from build123d import *

# Parameters (mm, degrees)
SKETCH_2_R               = 7.5
CUT_EXTRUDE_1_DEPTH      = 134.542128184
CUT_EXTRUDE_2_DEPTH      = 134.542128184
PATTERN_CIRCULAR_1_COUNT = 6
FILLET_1_R               = 2.5
SKETCH_4_R               = 100
SKETCH_4_R_2             = 72.5
CUT_EXTRUDE_3_DEPTH      = 20


with BuildPart() as part:
    # 草图1 → 旋转1 (revolve)
    with BuildSketch(Plane(origin=(0, 0, 0), x_dir=(0, 0, -1), z_dir=(1, 0, 0)), mode=Mode.PRIVATE) as revolve_1_sk:
        Polygon((-91.5, 33), (-91.5, 0), (-65, 0), (-65, 3), (-65, 33), (-69, 33), align=None)
    revolve(revolve_1_sk.sketch.rotate(Axis((0, 0, 0), (0, 1, 0)), 180), axis=Axis((0, 0, 0), (0, 1, 0)))

    # 草图2 → 切除-拉伸1 (cut, through all)
    with BuildSketch(Plane(origin=(0, 33, 0), x_dir=(1, 0, 0), z_dir=(0, 1, 0))):
        with Locations(Location((0, 80, 0), (0, 0, 270))):
            Circle(SKETCH_2_R)
    cut_extrude_1 = extrude(amount=-CUT_EXTRUDE_1_DEPTH, mode=Mode.SUBTRACT)

    # 草图3 → 切除-拉伸2 (cut, through all)
    with BuildSketch(Plane(origin=(0, 33, 0), x_dir=(1, 0, 0), z_dir=(0, 1, 0))):
        with BuildLine():
            Line((-72.788277417, 26.492766383), (-78.429157814, 28.545878943))
            ThreePointArc((-78.429157814, 28.545878943), (-80.374557913, 28.44634458), (-81.65798686, 26.980978151))
            ThreePointArc((-81.65798686, 26.980978151), (-86, 0), (-81.65798686, -26.980978151))
            ThreePointArc((-81.65798686, -26.980978151), (-80.374557913, -28.44634458), (-78.429157814, -28.545878943))
            Line((-78.429157814, -28.545878943), (-72.788277417, -26.492766383))
            ThreePointArc((-72.788277417, -26.492766383), (-71.394896395, -25.236492438), (-71.267736557, -23.364711127))
            ThreePointArc((-71.267736557, -23.364711127), (-75, 0), (-71.267736557, 23.364711127))
            ThreePointArc((-71.267736557, 23.364711127), (-71.394896395, 25.236492438), (-72.788277417, 26.492766383))
        make_face()
    cut_extrude_2 = extrude(amount=-CUT_EXTRUDE_2_DEPTH, mode=Mode.SUBTRACT)

    # 阵列(圆周)1: 切除-拉伸1, 切除-拉伸2 ×6 about axis
    pattern_circular_1_axis = Axis((0, 0, 0), (0, 1, 0))
    add([cut_extrude_1.rotate(pattern_circular_1_axis, i * 360 / PATTERN_CIRCULAR_1_COUNT) for i in range(1, PATTERN_CIRCULAR_1_COUNT)], mode=Mode.SUBTRACT)
    add([cut_extrude_2.rotate(pattern_circular_1_axis, i * 360 / PATTERN_CIRCULAR_1_COUNT) for i in range(1, PATTERN_CIRCULAR_1_COUNT)], mode=Mode.SUBTRACT)

    # 圆角1
    fillet_1_edges = [part.edges().sort_by_distance(p)[0] for p in [
        (0, 0, 65),
        (0, 0, 91.5),
    ]]
    fillet(fillet_1_edges, radius=FILLET_1_R)

    # 草图4 → 切除-拉伸3 (cut)
    with BuildSketch(Plane.XZ):
        Circle(SKETCH_4_R)
        with Locations(Location((0, 0, 0), (0, 0, 270))):
            Circle(SKETCH_4_R_2, mode=Mode.SUBTRACT)
    extrude(amount=-CUT_EXTRUDE_3_DEPTH, mode=Mode.SUBTRACT)


solid = part.part
For this review, take the finished solid that the model builds, in its own axes (mm). A direction names the side the tool comes from. Coordinates: 2 decimals unless noted, no trailing zeros. Loops run counter-clockwise (first coordinate to the right, second up) from the corner with the lowest first, then second, coordinate; pieces in that order, holes last. Notation, with made-up numbers: (1, 18) - (52, 18) arc R25 cw to (52, 37) - close; hole circle Ø5 at (71, 9.25). An arc over 180 degrees is marked (long way). Use a Markdown table: item, result. Add a question column.
Item 1: Insertion check: pin 1 Ø4 at (y, z) = (9, 5) entering from -X; pin 2 Ø8 at (x, y) = (67, 23) entering from -Z; pin 3 Ø4 at (x, y) = (-62, 24) entering from -Z. Each pin has a flat end and moves straight along its axis. Give the tip position at first contact, or say it passes through.
Item 2: Mouldability with a two-part tool opening along Z and no side actions: class faces 3 (the face through (48, 0, -48)), 4 (the face through (75, 27, 0)), 5 (the face through (13.98, 26.59, -79.28)) as pulls with the +Z half, pulls with the -Z half, needs draft (parallel to the pull), parting line crosses it, or undercut.
Item 3: For line 1 (X direction, y = 23, z = 40); line 2 (X direction, y = 26, z = -50.5); line 3 (Z direction, x = 50, y = 28), list the stretches that pass through material, from the lowest coordinate up.
Item 4: We need section B-B (y = 17). Give the boundary of the cut face in (x, z).
Item 5: Tool access review of faces 1 (the face through (75.648, 26.591, -27.534)), 2 (the face through (61, 33, 27)): name each direction out of +Z, -Z, +X, -X, +Y, -Y from which nothing blocks a thin tool from reaching the whole face with its end or side.
Item 6: We need section A-A (z = 0). Give the boundary of the cut face in (x, y).
Item 7: We need section D-D (z = -80). Give the boundary of the cut face in (x, y), and give its area (3 significant figures).
Item 8: We need section C-C (x = -4). Give the number of separate pieces and of enclosed holes in the cut face, and give its area (3 significant figures).
Results list:
| question | item | result |
|---|---|---|
| 1 | pin 1 | stops at x = -72.44 |
| 1 | pin 2 | stops at z = -66.36 |
| 1 | pin 3 | stops at z = -69.08 |
| 2 | face 3 | needs draft |
| 2 | face 4 | undercut |
| 2 | face 5 | undercut |
| 3 | line 1 | x = -82.29 to -76.78, -61.78 to -51.23, 51.23 to 61.78, 76.78 to 82.29 |
| 3 | line 2 | x = -76.3 to -60.18, -55.45 to -40.92, 40.92 to 55.45, 60.18 to 76.3 |
| 3 | line 3 | z = -76.63 to -69.97, -55.9 to -41.53, 41.53 to 55.9, 69.97 to 76.63 |
| 4 | outline | circle Ø145 at (0, 0); hole circle Ø130 at (0, 0) |
| 5 | face 1 | +Y, -Y |
| 5 | face 2 | +Z, -Z, +X, -X, +Y |
| 6 | outline | (-91.5, 20) - (-86, 20) - (-86, 33) - (-91.5, 33) - close; (-75, 20) - (-72.5, 20) - (-72.5, 0) - (-67.5, 0) arc R2.5 ccw to (-65, 2.5) - (-65, 33) - (-75, 33) - close; (65, 2.5) arc R2.5 ccw to (67.5, 0) - (72.5, 0) - (72.5, 20) - (75, 20) - (75, 33) - (65, 33) - close; (86, 20) - (91.5, 20) - (91.5, 33) - (86, 33) - close |
| 7 | outline | (-44.41, 20) - (-31.56, 20) - (-31.56, 33) - (-44.41, 33) - close; (-14.11, 20) - (-7.5, 20) - (-7.5, 33) - (-14.11, 33) - close; (7.5, 20) - (14.11, 20) - (14.11, 33) - (7.5, 33) - close; (31.56, 20) - (44.41, 20) - (44.41, 33) - (31.56, 33) - close |
| 7 | area | 506 mm^2 |
| 8 | separate pieces | 4 |
| 8 | enclosed holes | 0 |
| 8 | area | 658 mm^2 |
